Check sheet for the drawn part. Datum: minimum x, y, z corner. Units: mm. A direction names the side the tool comes from. Coordinates: 2 decimals unless noted, no trailing zeros. Write each loop counter-clockwise with the first axis right and the second up, starting at its lowest first coordinate (ties: lowest second). Pieces come first, ordered by that corner, then holes. Notation, with made-up numbers: (28, 33.25) -> (86, 33.25) arc R13 ccw to (86, 37.25) -> close; hole circle Ø6 at (0, -38.75). An arc over 180 degrees is marked (long way). Write item = value, one per line. Start each with the question number.
(1) Section check B-B (z = 125). Record the cut outline in (x, y), plus the area to 3 significant figures.
(2) Section check A-A (y = 6.5). Record the cut outline in (x, z), plus the area to 3 significant figures.
(3) Section check C-C (x = 103). Record the cut outline in (y, z), plus the area to 3 significant figures.
(4) Gauge pin test, flat ends, axial feed: pin 1 Ø4 at (y, z) = (29, 18.5) entering from -X; pin 2 Ø8 at (x, z) = (33, 129) entering from +Y. Record the tip position at first contact, or that the pin passes through.
(5) Mould release check, pull along X, two halves, no side actions. Record for the marked faces 1, 2 and 3: released by +X, released by -X, zero draft, split by the parting line, or undercut.
(6) Material ranges on probe 1 along Z at (x, y) = (74.5, 9); probe 2 along Y at (x, z) = (2, 115), recorded low to high. Write a range as [from, to].
(7) Set-up check for the marked faces 4 and 5: record each of +Z, -Z, +X, -X, +Y, -Y from which the full face is reachable in a straight line by a thin tool's end or side.
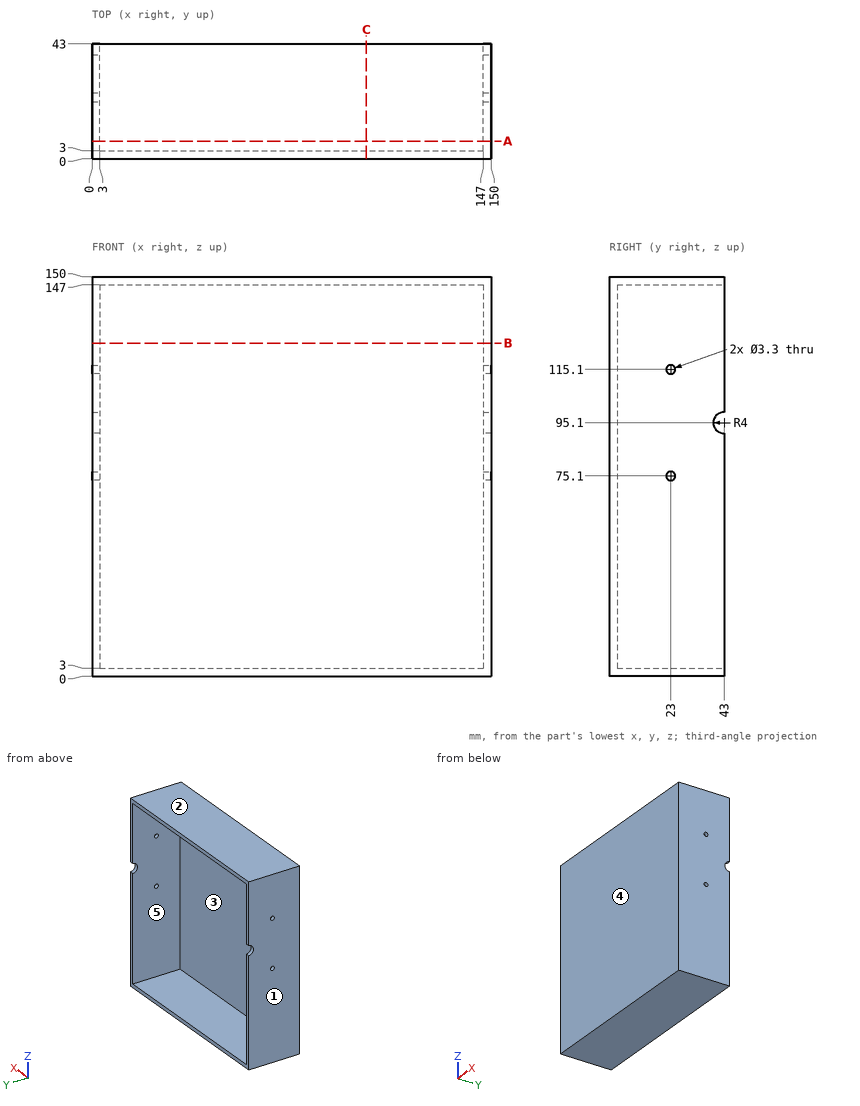
Response:
q1.outline = (0, 0) -> (150, 0) -> (150, 43) -> (147, 43) -> (147, 3) -> (3, 3) -> (3, 43) -> (0, 43) -> close
q1.area = 690 mm2
q2.outline = (0, 0) -> (150, 0) -> (150, 150) -> (0, 150) -> close; hole (3, 3) -> (147, 3) -> (147, 147) -> (3, 147) -> close
q2.area = 1,760 mm2
q3.outline = (0, 0) -> (43, 0) -> (43, 3) -> (3, 3) -> (3, 147) -> (43, 147) -> (43, 150) -> (0, 150) -> close
q3.area = 690 mm2
q4.pin_1 = 0
q4.pin_2 = 3
q5.face_1 = released by -X
q5.face_2 = zero draft
q5.face_3 = undercut
q6.probe_1 = [0, 3], [147, 150]
q6.probe_2 = [0, 21.35], [24.65, 43]
q7.face_4 = +Z, -Z, +X, -X, -Y
q7.face_5 = +Y
